Verification items for the finished model (mm, model axes). Round coordinates to 2 decimals unless told otherwise and drop trailing zeros. Write each loop counter-clockwise with the first axis right and the second up, starting at its lowest first coordinate (ties: lowest second). Pieces come first, ordered by that corner, then holes. Notation, with made-up numbers: M 61.5,31.25 L 85.5,31.25 A18 cw 85.5,36.25 Z; hole C 21,-25.75 d8. An arc over 180 degrees is marked long. One line per question, with ' | ' between items. Start each with the question number.
Q1. Cross-section at A-A (z = 30). Record the boundary of the cut face in (x, y).
Q2. Cross-section at C-C (x = 0). Record the boundary of the cut face in (y, z).
Q3. Gauge pin test, flat ends, axial feed: pin 1 (5.5 mm diameter, centred on x = -0.5, y = 4, fed in from -Z); pin 2 (1.8 mm diameter, centred on x = -0.5, y = 0.5, fed in from +Z); pin 3 (4 mm diameter, centred on x = -1, z = 85.5, fed in from -Y); pin 4 (5.5 mm diameter, centred on y = 3.5, z = 39.5, fed in from -X). Record the tip position at first contact, or that the pin passes through.
Q4. Cross-section at D-D (z = 97.5). Record the boundary of the cut face in (x, y), then the cut area to 3 significant figures.
Q5. Cross-section at B-B (y = 0). Record the boundary of the cut face in (x, z), then the cut area to 3 significant figures.
Q6. Thickness scan on line 1 along Y through (x, z) = (0, 173); line 2 along Z through (x, y) = (-0.5, -5.5); line 3 along X through (y, z) = (-6.75, 49). Record the ranges inside material, lowest first. Write a range as from..to.
from build123d import *

# Parameters (mm, degrees)
SKETCH1_R           = 10
BOSS_EXTRUDE1_DEPTH = 185
CUT_EXTRUDE1_DEPTH  = 70
SKETCH3_R           = 3
CUT_EXTRUDE2_DEPTH  = 20


with BuildPart() as part:
    # Sketch1 → Boss-Extrude1 (new body)
    with BuildSketch(Plane.XY):
        Circle(SKETCH1_R)
    extrude(amount=BOSS_EXTRUDE1_DEPTH)

    # Sketch1<3> → Cut-Extrude1 (cut)
    with BuildSketch(Plane.XY):
        with BuildLine():
            Line((3.5, -9.367496998), (3.5, 9.367496998))
            ThreePointArc((3.5, 9.367496998), (0, 10), (-3.5, 9.367496998))
            Line((-3.5, 9.367496998), (-3.5, -9.367496998))
            ThreePointArc((-3.5, -9.367496998), (0, -10), (3.5, -9.367496998))
        make_face()
    extrude(amount=CUT_EXTRUDE1_DEPTH, mode=Mode.SUBTRACT)

    # Sketch3 → Cut-Extrude2 (cut)
    with BuildSketch(Plane.XY.offset(185)):
        Circle(SKETCH3_R)
    extrude(amount=-CUT_EXTRUDE2_DEPTH, mode=Mode.SUBTRACT)


solid = part.part
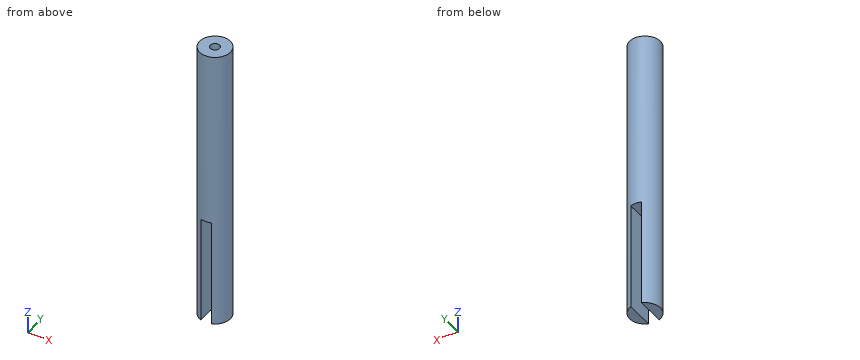
Determined:
1) outline: M -3.5,-9.37 L -3.5,9.37 A10 ccw Z; M 3.5,-9.37 A10 ccw 3.5,9.37 Z
2) outline: M -10,70 L 10,70 L 10,185 L 3,185 L 3,165 L -3,165 L -3,185 L -10,185 Z
3) pin 1: stops at z = 70 | pin 2: stops at z = 165 | pin 3: stops at y = -10 | pin 4: stops at x = -9.97
4) outline: C 0,0 d20 | area: 314 mm²
5) outline: M -10,0 L -3.5,0 L -3.5,70 L 3.5,70 L 3.5,0 L 10,0 L 10,185 L 3,185 L 3,165 L -3,165 L -3,185 L -10,185 Z | area: 3,090 mm²
6) line 1: y = -10..-3, 3..10 | line 2: z = 70..185 | line 3: x = -7.38..-3.5, 3.5..7.38
